Check sheet for the modelled part. Datum: model origin and axes. Units: mm. Round coordinates to 2 decimals unless told otherwise and drop trailing zeros. Loops run counter-clockwise (first coordinate to the right, second up) from the corner with the lowest first, then second, coordinate; pieces in that order, holes last. Notation, with made-up numbers: (-39.5, 51.25) - (-15.5, 51.25) arc R20 cw to (-15.5, 74.25) - close; hole circle Ø7 at (-27, 51.5). An arc over 180 degrees is marked (long way). Put each result on its own line as item: value.
```python
from build123d import *

# Parameters (mm, degrees)
F0_R            = 11.1
F1_DEPTH        = 7
F2_COUNT        = 3
F4_DEPTH        = 7
F4_COPIES_COUNT = 3


# Not quite as in the source:
# - a pattern or mirror of a feature is missing from the dataset's text; its kind, count and spacing are read off the source's solid


with BuildPart() as f1:
    # F0 (on Top) → F1 (new body)
    with BuildSketch(Plane.XY):
        with BuildLine():
            ThreePointArc((-9.612881982, 5.55), (0, 11.1), (9.612881982, 5.55))
            Line((9.612881982, 5.55), (12.2109581934, 7.05))
            ThreePointArc((12.2109581934, 7.05), (10.0807621135, 15), (12.2109581934, 22.95))
            ThreePointArc((12.2109581934, 22.95), (0, 44.1), (-12.2109581934, 22.95))
            ThreePointArc((-12.2109581934, 22.95), (-10.0807621135, 15), (-12.2109581934, 7.05))
            Line((-12.2109581934, 7.05), (-9.612881982, 5.55))
        make_face()
        with Locations((0, 30)):
            Circle(F0_R, mode=Mode.SUBTRACT)
    extrude(amount=F1_DEPTH)

    # F2: F1 ×3 about axis
    f2_axis = Axis((0, 0, 0), (0, 0, 1))


with BuildPart() as f1_1:
    add(f1.part)
    for i in range(1, F2_COUNT):
        add(f1.part.rotate(f2_axis, i * 360 / F2_COUNT))

    # F3 (on face) → F4 (join)
    with BuildSketch(Plane.XY):
        with BuildLine():
            Line((36.8595294383, -6.0299151903), (40.0530223584, -15.8840201358))
            ThreePointArc((40.0530223584, -15.8840201358), (31.9933329124, 18.4713593692), (6.2705462274, 42.6289449286))
            ThreePointArc((6.2705462274, 42.6289449286), (10.4711494103, 39.4427236552), (13.2077049817, 34.9362464602))
            ThreePointArc((13.2077049817, 34.9362464602), (29.395256701, 16.9713593692), (36.8595294383, -6.0299151903))
        make_face()
    f4 = extrude(amount=F4_DEPTH)

    # F4_copies: F4 ×3 about axis
    f4_copies_axis = Axis((0, 0, 0), (0, 0, 1))
    for i in range(1, F4_COPIES_COUNT):
        add(f4.rotate(f4_copies_axis, i * 360 / F4_COPIES_COUNT))


solid = f1_1.part
```
Item 1: Section check A-A on y = 30. Enter the section's corners in (x, z), then the cut area to 3 significant figures.
Filled sheet:
outline: (-23.38, 0) - (-19.14, 0) - (-19.14, 7) - (-23.38, 7) - close; (-14.1, 0) - (-11.1, 0) - (-11.1, 7) - (-14.1, 7) - close; (11.1, 0) - (14.1, 0) - (14.1, 7) - (11.1, 7) - close; (19.14, 0) - (23.38, 0) - (23.38, 7) - (19.14, 7) - close
area: 101 mm²
Item 2: Release check for a two-part mould opening along Y. For faces 1 (the cylindrical face through (-0.5, -36.94, 3.45)), 2 (the flat face through (-10, 6, 0)), 3 (the cylindrical face through (0.1, 44.1, 3.5)), 4 (the cylindrical face through (10.6, 33.3, 3.5)) record: +Y half, -Y half, draft (parallel to the pull), parting line (faces both ways), or undercut.
Filled sheet:
face 1: -Y half
face 2: draft
face 3: +Y half
face 4: undercut
Item 3: Section check B-B on z = 5.75. Enter the section's corners in (x, y).
Filled sheet:
outline: (-40.05, -15.88) arc R14.1 ccw to (-33.78, -26.74) arc R61.05 ccw to (33.78, -26.74) arc R14.1 ccw to (40.05, -15.88) arc R61.05 ccw to (6.27, 42.63) arc R14.1 ccw to (-6.27, 42.63) arc R61.05 ccw to start; hole circle Ø22.2 at (-25.98, -15); hole (-36.86, -6.03) arc R14.1 cw to (-25.98, -0.9) arc R15.9 ccw to (-12.21, 22.95) arc R14.1 cw to (-13.21, 34.94) arc R58.05 ccw to start; hole (-23.65, -28.91) arc R58.05 ccw to (23.65, -28.91) arc R14.1 cw to (13.77, -22.05) arc R15.9 ccw to (-13.77, -22.05) arc R14.1 cw to start; hole circle Ø22.2 at (0, 0); hole circle Ø22.2 at (0, 30); hole (12.21, 22.95) arc R15.9 ccw to (25.98, -0.9) arc R14.1 cw to (36.86, -6.03) arc R58.05 ccw to (13.21, 34.94) arc R14.1 cw to start; hole circle Ø22.2 at (25.98, -15)
Item 4: Go/stop test with flat-tipped pins: pin 1 (4 mm diameter, centred on x = 18.5, y = -22.5, fed in from +Z); pin 2 (2 mm diameter, centred on x = 31, z = 4.5, fed in from -Y); pin 3 (2 mm diameter, centred on y = -15.5, z = 6, fed in from -X); pin 4 (1 mm diameter, centred on y = 2.5, z = 5.5, fed in from +X). Record where each tip stops, or that it passes through.
Filled sheet:
pin 1: z = 7
pin 2: y = -29.06
pin 3: x = -40.12
pin 4: x = 38.53
Item 5: Thickness scan on line 1 (Y direction, x = 16, z = 6); line 2 (X direction, y = -21.5, z = 2.25); line 3 (X direction, y = -13, z = 3.5). Record the ranges inside material, lowest first. Write a range as from..to.
Filled sheet:
line 1: -34.81..-31.69, -24.96..-19.86, -10.14..2.62, 32.78..36.6
line 2: -38.49..-34.98, -16.98..-13.44, 13.44..16.98, 34.98..38.49
line 3: -40.17..-36.9, -15.06..15.06, 36.9..40.17
Item 6: Section check C-C on x = 30.5. Enter the section's corners in (y, z).
Filled sheet:
outline: (-28.78, 0) - (-25.14, 0) - (-25.14, 7) - (-28.78, 7) - close; (-4.86, 0) - (-1.64, 0) - (-1.64, 7) - (-4.86, 7) - close; (14.97, 0) - (20.92, 0) - (20.92, 7) - (14.97, 7) - close
Item 7: Section check D-D on x = -1.5. Enter the section's corners in (y, z).
Filled sheet:
outline: (-36.92, 0) - (-33.92, 0) - (-33.92, 7) - (-36.92, 7) - close; (-14.17, 0) - (-11, 0) - (-11, 7) - (-14.17, 7) - close; (11, 0) - (19, 0) - (19, 7) - (11, 7) - close; (41, 0) - (44.02, 0) - (44.02, 7) - (41, 7) - close
